from build123d import *

# Parameters (mm, degrees)
BOSS_EXTRUDE1_DEPTH            = 25
BOSS_EXTRUDE2_DEPTH            = 50
BOSS_EXTRUDE2_DEPTH_BACK       = 22
CUT_EXTRUDE1_DEPTH             = 89.177744216
CUT_EXTRUDE1_DEPTH_BACK        = 89.177744216
SKETCH3_R                      = 4
SKETCH4_R                      = 6
CUT_EXTRUDE2_DEPTH             = 2
CUT_EXTRUDE3_DEPTH             = 77.421950872
CUT_EXTRUDE3_DEPTH_BACK        = 77.421950872
F_2_3_2_3_DIAMETER_HOLE1_D     = 2.3
F_2_3_2_3_DIAMETER_HOLE1_DEPTH = 4
F_2_3_2_3_DIAMETER_HOLE1_TIP   = 0.690989712


with BuildPart() as part:
    # Sketch1 → Boss-Extrude1 (new, symmetric)
    with BuildSketch(Plane(origin=(0, 0, 0), x_dir=(0, 0, -1), z_dir=(1, 0, 0))):
        with BuildLine():
            Line((0, 0), (-40.343145751, 0))
            ThreePointArc((-40.343145751, 0), (-44.038663881, 2.469266271), (-43.171572875, 6.828427125))
            Line((-43.171572875, 6.828427125), (-15, 35))
            Line((-15, 35), (0, 35))
            Line((0, 35), (0, 0))
        make_face()
    extrude(amount=BOSS_EXTRUDE1_DEPTH, both=True)

    # Sketch2 → Boss-Extrude2 (add, two sides: drawn at the far end of the back side and taken through both)
    with BuildSketch(Plane(origin=(0, 0, 0), x_dir=(1, 0, 0), z_dir=(0, 1, 0)).offset(-BOSS_EXTRUDE2_DEPTH_BACK)):
        with BuildLine():
            Line((-7.794228634, -13.5), (-13.856406461, -24))
            ThreePointArc((-13.856406461, -24), (-14.124355653, -25), (-13.856406461, -26))
            Line((-13.856406461, -26), (-7.794228634, -36.5))
            ThreePointArc((-7.794228634, -36.5), (-7.062177826, -37.232050808), (-6.062177826, -37.5))
            Line((-6.062177826, -37.5), (6.062177826, -37.5))
            ThreePointArc((6.062177826, -37.5), (7.062177826, -37.232050808), (7.794228634, -36.5))
            Line((7.794228634, -36.5), (13.856406461, -26))
            ThreePointArc((13.856406461, -26), (14.124355653, -25), (13.856406461, -24))
            Line((13.856406461, -24), (7.794228634, -13.5))
            ThreePointArc((7.794228634, -13.5), (7.062177826, -12.767949192), (6.062177826, -12.5))
            Line((6.062177826, -12.5), (-6.062177826, -12.5))
            ThreePointArc((-6.062177826, -12.5), (-7.062177826, -12.767949192), (-7.794228634, -13.5))
        make_face()
    extrude(amount=BOSS_EXTRUDE2_DEPTH + BOSS_EXTRUDE2_DEPTH_BACK)

    # Sketch3 → Cut-Extrude1 (cut, two sides: drawn at the far end of the back side and taken through both)
    with BuildSketch(Plane(origin=(0, 50, 0), x_dir=(1, 0, 0), z_dir=(0, 1, 0)).offset(-CUT_EXTRUDE1_DEPTH_BACK)):
        with Locations(Location((0, -25, 0), (0, 0, 270))):
            Circle(SKETCH3_R)
    extrude(amount=CUT_EXTRUDE1_DEPTH + CUT_EXTRUDE1_DEPTH_BACK, mode=Mode.SUBTRACT)

    # Sketch4 → Cut-Extrude2 (cut)
    with BuildSketch(Plane(origin=(0, 50, 0), x_dir=(1, 0, 0), z_dir=(0, 1, 0))):
        with Locations(Location((0, -25, 0), (0, 0, 270))):
            Circle(SKETCH4_R)
    extrude(amount=-CUT_EXTRUDE2_DEPTH, mode=Mode.SUBTRACT)

    # Sketch5 → Cut-Extrude3 (cut, two sides: drawn at the far end of the back side and taken through both)
    with BuildSketch(Plane(origin=(0, 35, 0), x_dir=(1, 0, 0), z_dir=(0, 1, 0)).offset(-CUT_EXTRUDE3_DEPTH_BACK)):
        Polygon((-17.594174213, -7.5), (17.594174213, -7.5), (16, 0), (-16, 0), align=None)
    extrude(amount=CUT_EXTRUDE3_DEPTH + CUT_EXTRUDE3_DEPTH_BACK, mode=Mode.SUBTRACT)

    # Ø2.3 (2.3) Diameter Hole1
    with Locations(Plane(origin=(0, 50, 0), x_dir=(1, 0, 0), z_dir=(0, 1, 0))):
        with Locations((-11.547005384, -25), (-5.773502692, -15), (5.773502692, -15), (11.547005384, -25), (5.773502692, -35), (-5.773502692, -35)):
            Hole(F_2_3_2_3_DIAMETER_HOLE1_D / 2, depth=F_2_3_2_3_DIAMETER_HOLE1_DEPTH)
            with Locations((0, 0, -(F_2_3_2_3_DIAMETER_HOLE1_DEPTH + F_2_3_2_3_DIAMETER_HOLE1_TIP / 2))):  # 118° drill point
                Cone(0, F_2_3_2_3_DIAMETER_HOLE1_D / 2, F_2_3_2_3_DIAMETER_HOLE1_TIP, mode=Mode.SUBTRACT)


solid = part.part
Build history of the part. All positions in model axes, mm. A direction names the side the tool comes from. Coordinates: 2 decimals unless noted, no trailing zeros. Order: outer loops, then holes, each group sorted by start corner. A loop starts at its lowest first (then second) coordinate and runs counter-clockwise, first axis right, second up. Notation, with made-up numbers: (33.25, 77) - (60.25, 77) arc R19 cw to (60.25, 104) - close; hole circle Ø7 at (54.5, -14). An arc over 180 degrees is marked (long way). Write item = value, one per line. Start each with the question number.
1) Two-plate mould, pull along Z, no slides. Class faces 5 (the face through (0, -11, 12.5)), 6 (the face through (5.964, 45.429, 14.94)), 7 (the face through (10.783, 35.55, 31.324)), 8 (the face through (-5.921, 45.429, 14.865)): pulls with the +Z half, pulls with the -Z half, needs draft (parallel to the pull), parting line crosses it, or undercut.
2) Saw through at C-C on y = 43. Write the cut outline in (x, z).
3) Flat gauge pins, fed straight in: pin 1 Ø8 at (y, z) = (-3, 6) entering from -X; pin 2 Ø1 at (y, z) = (26.5, 39) entering from -X; pin 3 Ø3.5 at (x, y) = (-1.5, 42) entering from -Z; pin 4 Ø9.5 at (x, y) = (-0.5, 36.5) entering from +Z. Where does each tip first touch, or does it go through?
4) Saw through at B-B on y = 25. Write the cut outline in (x, z).
5) Saw through at A-A on x = 0. Write the cut outline in (y, z).
6) 3-axis set-ups, long thin cutter, end or side, ignore diameter. For faces 1 (the face through (-5.52, 47.97, 36.12)), 2 (the face through (0, 42, 12.5)), 3 (the face through (-10.783, -11.154, 18.676)), 4 (the face through (-7.075, 30.987, 37.225)): which of +Z, -Z, +X, -X, +Y, -Y reach the whole face in a straight line?
7) Wall check: line 1 along X through (y, z) = (48.5, 25); line 2 along X through (y, z) = (47.7, 15); line 3 along X through (y, z) = (-17.5, 25). Give the ranges that are in metal, low to high. Write a range as from..to.
From the geometry:
q1.face_5 = pulls with the -Z half
q1.face_6 = undercut
q1.face_7 = pulls with the +Z half
q1.face_8 = undercut
q2.outline = (-13.86, 24) - (-7.79, 13.5) arc R2 ccw to (-6.06, 12.5) - (6.06, 12.5) arc R2 ccw to (7.79, 13.5) - (13.86, 24) arc R2 ccw to (13.86, 26) - (7.79, 36.5) arc R2 ccw to (6.06, 37.5) - (-6.06, 37.5) arc R2 ccw to (-7.79, 36.5) - (-13.86, 26) arc R2 ccw to start; hole circle Ø8 at (0, 25)
q3.pin_1 = -25
q3.pin_2 = through
q3.pin_3 = 12.5
q3.pin_4 = 37.5
q4.outline = (-25, 0) - (-16, 0) - (-17.59, 7.5) - (17.59, 7.5) - (16, 0) - (25, 0) - (25, 25) - (14.12, 25) arc R2 ccw to (13.86, 26) - (7.79, 36.5) arc R2 ccw to (6.06, 37.5) - (-6.06, 37.5) arc R2 ccw to (-7.79, 36.5) - (-13.86, 26) arc R2 ccw to (-14.12, 25) - (-25, 25) - close; hole circle Ø8 at (0, 25)
q5.outline = (-22, 12.5) - (0, 12.5) - (0, 7.5) - (35, 7.5) - (35, 12.5) - (50, 12.5) - (50, 19) - (48, 19) - (48, 21) - (-22, 21) - close; (-22, 29) - (48, 29) - (48, 31) - (50, 31) - (50, 37.5) - (12.5, 37.5) - (6.83, 43.17) arc R4 ccw to (0, 40.34) - (0, 37.5) - (-22, 37.5) - close
q6.face_1 = +Y
q6.face_2 = -Z, +X, -X, +Y
q6.face_3 = -Z, -X, -Y
q6.face_4 = +Z, -X, +Y
q7.line_1 = -14.12..-12.7, -10.4..-6, 6..10.4, 12.7..14.12
q7.line_2 = -8.66..-6.92, -4.62..4.62, 6.92..8.66
q7.line_3 = -14.12..-4, 4..14.12
